```python
from build123d import *

# Parameters (mm, degrees)
SKETCH1_W           = 26.5
SKETCH1_H           = 37.5
BOSS_EXTRUDE1_DEPTH = 4.353
SKETCH2_W           = 23.4
SKETCH2_H           = 34.9
CUT_EXTRUDE1_DEPTH  = 1.6
SKETCH3_W           = 1.55
SKETCH3_H           = 13
CUT_EXTRUDE2_DEPTH  = 1.6
SKETCH4_W           = 2.753
SKETCH4_H           = 13
CUT_EXTRUDE3_DEPTH  = 1
SKETCH5_W           = 1.55
SKETCH5_H           = 9.5
CUT_EXTRUDE5_DEPTH  = 1.6
CUT_EXTRUDE6_DEPTH  = 9.5
SKETCH7_W           = 4.587747781
SKETCH7_H           = 26.668615153
SKETCH7_W_2         = 9.921470812
SKETCH7_H_2         = 17.49311959
CUT_EXTRUDE7_DEPTH  = 2
SKETCH8_W           = 1.6
SKETCH8_H           = 3.8
BOSS_EXTRUDE2_DEPTH = 1.6


with BuildPart() as part:
    # Sketch1 → Boss-Extrude1 (new body)
    with BuildSketch(Plane.YZ):
        with Locations((57.87, 107.93)):
            Rectangle(SKETCH1_W, SKETCH1_H)
    extrude(amount=BOSS_EXTRUDE1_DEPTH)

    # Sketch2 → Cut-Extrude1 (cut)
    with BuildSketch(Plane.YZ.offset(4.353)):
        with Locations((57.87, 107.93)):
            Rectangle(SKETCH2_W, SKETCH2_H)
    extrude(amount=-CUT_EXTRUDE1_DEPTH, mode=Mode.SUBTRACT)

    # Sketch3 → Cut-Extrude2 (cut)
    with BuildSketch(Plane.YZ.offset(4.353)):
        with Locations((45.395, 107.93)):
            Rectangle(SKETCH3_W, SKETCH3_H)
    extrude(amount=-CUT_EXTRUDE2_DEPTH, mode=Mode.SUBTRACT)

    # Sketch4 → Cut-Extrude3 (cut)
    with BuildSketch(Plane.XZ.offset(-44.62)):
        with Locations((1.3765, 107.93)):
            Rectangle(SKETCH4_W, SKETCH4_H)
    extrude(amount=-CUT_EXTRUDE3_DEPTH, mode=Mode.SUBTRACT)

    # Sketch5 → Cut-Extrude5 (cut)
    with BuildSketch(Plane.YZ.offset(4.353)):
        with Locations((45.395, 93.93)):
            Rectangle(SKETCH5_W, SKETCH5_H)
    extrude(amount=-CUT_EXTRUDE5_DEPTH, mode=Mode.SUBTRACT)

    # Sketch6 → Cut-Extrude6 (cut)
    with BuildSketch(Plane(origin=(0, 0, 89.18), x_dir=(1, 0, 0), z_dir=(0, 0, -1))):
        Polygon((1.953, -46.17), (2.753, -46.17), (2.753, -44.62), (0, -44.62), (0, -49.12), (1.953, -49.12), align=None)
    extrude(amount=-CUT_EXTRUDE6_DEPTH, mode=Mode.SUBTRACT)

    # Sketch7 → Cut-Extrude7 (cut)
    with BuildSketch(Plane(origin=(0, 0, 0), x_dir=(0, -1, 0), z_dir=(-1, 0, 0))):
        with Locations((-52.536232928, 109.172253496)):
            Rectangle(SKETCH7_W, SKETCH7_H)
        Polygon((-57.329123903, 95.837945919), (-57.329123903, 90.653417938), (-49.12, 90.653417938), (-49.12, 95.837945919), (-50.242359038, 95.837945919), (-54.830106819, 95.837945919), align=None)
        with Locations((-61.879572923, 107.531107948)):
            Rectangle(SKETCH7_W_2, SKETCH7_H_2)
    extrude(amount=-CUT_EXTRUDE7_DEPTH, mode=Mode.SUBTRACT)

    # Sketch8 → Boss-Extrude2 (add)
    with BuildSketch(Plane(origin=(0, 0, 0), x_dir=(0, -1, 0), z_dir=(-1, 0, 0))):
        with Locations((-68.22, 123.18)):
            Rectangle(SKETCH8_W, SKETCH8_H)
    boss_extrude2 = extrude(amount=BOSS_EXTRUDE2_DEPTH)

    # Mirror1: Boss-Extrude2 across plane
    add(boss_extrude2.mirror(Plane(origin=(0, 0, 107.93), x_dir=(1, 0, 0), z_dir=(0, 0, -1))))

    # Mirror2: Boss-Extrude2 across plane
    add(boss_extrude2.mirror(Plane(origin=(0, 57.62, 0), x_dir=(0, 0, 1), z_dir=(0, -1, 0))))


solid = part.part
```
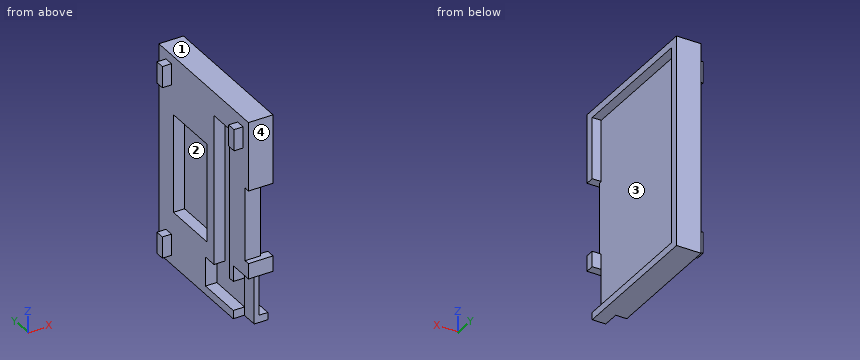
Read the model definition and answer for the solid it produces. Units are mm, in the model's axes. Face numbers are marked on the shaded views. Coordinates: 2 decimals unless noted, no trailing zeros. Order: outer loops, then holes, each group sorted by start corner. A loop starts at its lowest first (then second) coordinate and runs counter-clockwise, first axis right, second up. Notation, with made-up numbers: (6, 22) - (25, 22) arc R17 ccw to (25, 49) - close; hole circle Ø2 at (-27, 30). An arc over 180 degrees is marked (long way). Answer as a JSON object with one key per item and string values. Group by question number.
Item 1: Consider probe 1 along Y at (x, z) = (1.6, 114); probe 2 along Z at (x, y) = (1.1, 61.25); probe 3 along Z at (x, y) = (-1.1, 68). Determine where each line is inside the solid, lowest interval first. Write a range as from..to.
Item 2: Section B-B (y = 54) is taken. Give the vertices of the cut face in (x, z), plus the area to 3 significant figures.
Item 3: The mould has two halves that part along Z. Classify the marked faces 1, 2, 3 and 4: +Z half, -Z half, draft (parallel to the pull), parting line (faces both ways), or undercut.
Item 4: Section D-D (x = 0.95) is taken. Give the vertices of the cut face in (y, z), plus the area to 3 significant figures.
Item 5: Section A-A (x = 3.6) is taken. Give the vertices of the cut face in (y, z), plus the area to 3 significant figures.
Item 6: Flat-ended cylindrical pins translate along their axes: P1, Ø10, axis at y = 53, z = 107.5, coming from the -X side; P2, Ø6, axis at y = 51, z = 117, coming from the +X side; P3, Ø1.3, axis at x = -1, y = 68, coming from the -Z side. Find the tip coordinate at first contact, or state that the pin passes through.
Item 7: Section C-C (z = 94) is taken. Give the vertices of the cut face in (x, y), plus the area to 3 significant figures.
Results are:
{
 "1": {"probe 1": "y = 45.62..50.24, 54.83..56.92, 66.84..71.12", "probe 2": "z = 89.18..98.78, 116.28..126.68", "probe 3": "z = 90.78..94.58, 121.28..125.08"},
 "2": {"outline": "(0, 89.18) - (4.35, 89.18) - (4.35, 90.48) - (2.75, 90.48) - (2.75, 125.38) - (4.35, 125.38) - (4.35, 126.68) - (0, 126.68) - (0, 122.51) - (2, 122.51) - (2, 90.65) - (0, 90.65) - close", "area": "43.7 mm^2"},
 "3": {"face 1": "+Z half", "face 2": "undercut", "face 3": "undercut", "face 4": "draft"},
 "4": {"outline": "(44.62, 98.68) - (49.12, 98.68) - (49.12, 95.84) - (50.24, 95.84) - (50.24, 122.51) - (54.83, 122.51) - (54.83, 95.84) - (57.33, 95.84) - (57.33, 90.65) - (49.12, 90.65) - (49.12, 89.18) - (71.12, 89.18) - (71.12, 126.68) - (44.62, 126.68) - (44.62, 114.43) - (45.62, 114.43) - (45.62, 101.43) - (44.62, 101.43) - close; hole (56.92, 98.78) - (66.84, 98.78) - (66.84, 116.28) - (56.92, 116.28) - close", "area": "600 mm^2"},
 "5": {"outline": "(44.62, 98.68) - (46.17, 98.68) - (46.17, 101.43) - (44.62, 101.43) - close; (44.62, 114.43) - (46.17, 114.43) - (46.17, 125.38) - (69.57, 125.38) - (69.57, 90.48) - (46.17, 90.48) - (46.17, 89.18) - (71.12, 89.18) - (71.12, 126.68) - (44.62, 126.68) - close", "area": "142 mm^2"},
 "6": {"P1": "stops at x = 0", "P2": "stops at x = 2.75", "P3": "stops at z = 90.78"},
 "7": {"outline": "(-1.6, 67.42) - (0, 67.42) - (0, 57.33) - (2, 57.33) - (2, 49.12) - (1.95, 49.12) - (1.95, 46.17) - (2.75, 46.17) - (2.75, 69.57) - (4.35, 69.57) - (4.35, 71.12) - (0, 71.12) - (0, 69.02) - (-1.6, 69.02) - close", "area": "51.5 mm^2"}
}
